```python
from build123d import *

# Parameters (mm, degrees)
F0_W     = 50.8
F0_H     = 50.8
F1_DEPTH = 43.434
F2_W     = 12.192
F2_H     = 12.192
F3_DEPTH = 17.78
F4_W     = 12.192
F4_H     = 12.192
F5_DEPTH = 17.78


with BuildPart() as f1:
    # F0 (on Front) → F1 (new body)
    with BuildSketch(Plane.XZ):
        with Locations((0.816428, 3.06024)):
            Rectangle(F0_W, F0_H)
    extrude(amount=F1_DEPTH)

    # F2 (on face) → F3 (cut)
    with BuildSketch(Plane(origin=(0, 0, 0), x_dir=(-1, 0, 0), z_dir=(0, 1, 0))):
        with Locations((-16.600084, 18.591136)):
            Rectangle(F2_W, F2_H)
    extrude(amount=-F3_DEPTH, mode=Mode.SUBTRACT)

    # F4 (on face) → F5 (cut)
    with BuildSketch(Plane(origin=(0, 0, 0), x_dir=(-1, 0, 0), z_dir=(0, 1, 0))):
        with Locations((0.544286, 18.74946)):
            Rectangle(F4_W, F4_H)
    extrude(amount=-F5_DEPTH, mode=Mode.SUBTRACT)


solid = f1.part
```
Work out the finished part from the listing and answer in its coordinate system (mm). A direction names the side the tool comes from. Coordinates: 2 decimals unless noted, no trailing zeros. Loops run counter-clockwise (first coordinate to the right, second up) from the corner with the lowest first, then second, coordinate; pieces in that order, holes last. Notation, with made-up numbers: M -33,-17 L 2,-17 A30 cw 2,5 Z; hole C 7,-9 d9. An arc over 180 degrees is marked long. Use CSV: the item, a comma, the result in double quotes. Start each with the question number.
(1) Find section B-B, the plane z = 24. Give the vertices of the cut face in (x, y), then the cut area to 3 significant figures.
(2) Find section C-C, the plane x = 20.5. Give the vertices of the cut face in (y, z), then the cut area to 3 significant figures.
(3) For faces 1 (the face through (17, -9, 24.687)), 2 (the face through (26.216, -21, 3)), determine the directions among +Z, -Z, +X, -X, +Y, -Y from which every point of the face is accessible in a straight line to the end or side of a thin tool.
(4) For a pull along Z with two mould halves and no side action, classify faces 3 (the face through (0, -21, 28.46)), 4 (the face through (0, -9, 12.653)), 5 (the face through (-24.584, -21, 3)) as +Z half, -Z half, draft (parallel to the pull), parting line (faces both ways), or undercut.
(5) Consider line 1 (X direction, y = -5, z = 17.5); line 2 (Z direction, x = -5, y = -3); line 3 (Z direction, x = 13, y = -16.5). Determine where each line is inside the solid, lowest interval first.
(6) Find section A-A, the plane y = -4. Give the vertices of the cut face in (x, z), then the cut area to 3 significant figures.
Recorded:
1,outline,"M -24.58,-43.43 L 26.22,-43.43 L 26.22,0 L 22.7,0 L 22.7,-17.78 L 10.5,-17.78 L 10.5,0 L 5.55,0 L 5.55,-17.78 L -6.64,-17.78 L -6.64,0 L -24.58,0 Z"
1,area,"1,770 mm^2"
2,outline,"M -43.43,-22.34 L 0,-22.34 L 0,12.5 L -17.78,12.5 L -17.78,24.69 L 0,24.69 L 0,28.46 L -43.43,28.46 Z"
2,area,"1,990 mm^2"
3,face 1,"+Y"
3,face 2,"+Z, -Z, +X, +Y, -Y"
4,face 3,"+Z half"
4,face 4,"undercut"
4,face 5,"draft"
5,line 1,"x = -24.58 to -6.64, 5.55 to 10.5, 22.7 to 26.22"
5,line 2,"z = -22.34 to 12.65, 24.85 to 28.46"
5,line 3,"z = -22.34 to 12.5, 24.69 to 28.46"
6,outline,"M -24.58,-22.34 L 26.22,-22.34 L 26.22,28.46 L -24.58,28.46 Z; hole M -6.64,12.65 L 5.55,12.65 L 5.55,24.85 L -6.64,24.85 Z; hole M 10.5,12.5 L 22.7,12.5 L 22.7,24.69 L 10.5,24.69 Z"
6,area,"2,280 mm^2"
